```python
from build123d import *
from build123d.topology import SkipClean

# Parameters (mm, degrees)
SKETCH1_R                       = 246.38
SKETCH1_R_2                     = 59.69
BOSS_EXTRUDE1_DEPTH             = 81.28
SKETCH2_R                       = 355.6
SKETCH2_R_2                     = 246.38
BOSS_EXTRUDE2_DEPTH             = 204.47
BOSS_EXTRUDE3_START             = 381
SKETCH3_R                       = 254
BOSS_EXTRUDE3_DEPTH             = 25.4
BOSS_EXTRUDE3_DIRECTION_2_REACH = 1339.721
SKETCH4_R                       = 30.48
CUT_EXTRUDE1_DEPTH              = 38.1
SKETCH4_4_R                     = 127
CUT_EXTRUDE2_DEPTH              = 63.5
SKETCH5_R                       = 71.12
CUT_EXTRUDE3_DEPTH              = 762


with BuildPart() as part:
    # Sketch1 → Boss-Extrude1 (new body)
    with BuildSketch(Plane(origin=(0, 0, 0), x_dir=(1, 0, 0), z_dir=(0, 1, 0))):
        with BuildLine():
            Line((-127, 444.5), (-127, 332.148099))
            ThreePointArc((-127, 332.148099), (-307.958634, 177.8), (-351.148692, -56.088823))
            Line((-351.148692, -56.088823), (-448.448292, -112.264774))
            ThreePointArc((-448.448292, -112.264774), (-494.933518, -285.75), (-321.448292, -332.235226))
            Line((-321.448292, -332.235226), (-224.148692, -276.059276))
            ThreePointArc((-224.148692, -276.059276), (0, -355.6), (224.148692, -276.059276))
            Line((224.148692, -276.059276), (321.448292, -332.235226))
            ThreePointArc((321.448292, -332.235226), (494.933518, -285.75), (448.448292, -112.264774))
            Line((448.448292, -112.264774), (351.148692, -56.088823))
            ThreePointArc((351.148692, -56.088823), (307.958634, 177.8), (127, 332.148099))
            Line((127, 332.148099), (127, 444.5))
            ThreePointArc((127, 444.5), (0, 571.5), (-127, 444.5))
        make_face()
        with Locations(Location((0, 0, 0), (0, 0, 270))):
            Circle(SKETCH1_R, mode=Mode.SUBTRACT)
        with Locations(Location((0, 444.5, 0), (0, 0, 270))):
            Circle(SKETCH1_R_2, mode=Mode.SUBTRACT)
        with Locations(Location((384.948292, -222.25, 0), (0, 0, 270))):
            Circle(SKETCH1_R_2, mode=Mode.SUBTRACT)
        with Locations(Location((-384.948292, -222.25, 0), (0, 0, 270))):
            Circle(SKETCH1_R_2, mode=Mode.SUBTRACT)
    extrude(amount=BOSS_EXTRUDE1_DEPTH)

    # Sketch2 → Boss-Extrude2 (add)
    with BuildSketch(Plane(origin=(0, 81.28, 0), x_dir=(1, 0, 0), z_dir=(0, 1, 0))):
        with Locations(Location((0, 0, 0), (0, 0, 69.075168))):
            Circle(SKETCH2_R)
        with Locations(Location((0, 0, 0), (0, 0, 270))):
            Circle(SKETCH2_R_2, mode=Mode.SUBTRACT)
    extrude(amount=BOSS_EXTRUDE2_DEPTH)

    # Mirror2: part across plane


with BuildPart() as part_1:
    add(part.part)
    add(part.part.mirror(Plane.ZX.offset(285.75)))

    # Sketch3 → Boss-Extrude3 (add)
    with BuildSketch(Plane.XY.offset(BOSS_EXTRUDE3_START)):
        with Locations((0, 285.75)):
            Circle(SKETCH3_R)
    extrude(amount=BOSS_EXTRUDE3_DEPTH)

    # Sketch3 → Boss-Extrude3 direction 2 (add, up to next)
    with BuildSketch(Plane.XY.offset(BOSS_EXTRUDE3_START), mode=Mode.PRIVATE) as boss_extrude3_direction_2_sk1:
        with Locations((0, 285.75)):
            Circle(SKETCH3_R)
    boss_extrude3_direction_2_tool1 = extrude(boss_extrude3_direction_2_sk1.sketch, amount=-BOSS_EXTRUDE3_DIRECTION_2_REACH, mode=Mode.PRIVATE) - part_1.part
    add(boss_extrude3_direction_2_tool1.solids().sort_by_distance((0, 285.75, 381))[0])

    # Sketch4 → Cut-Extrude1 (cut)
    with SkipClean():  # the faces are left unmerged after this step: merging them gives an invalid solid
        with BuildSketch(Plane.XY.offset(406.4)):
            with Locations((0, 476.25)):
                Circle(SKETCH4_R)
            with Locations((164.977839, 190.5)):
                Circle(SKETCH4_R)
            with Locations((-164.977839, 190.5)):
                Circle(SKETCH4_R)
        extrude(amount=-CUT_EXTRUDE1_DEPTH, mode=Mode.SUBTRACT)

    # Sketch4_4 → Cut-Extrude2 (cut)
    with SkipClean():  # the faces are left unmerged after this step: merging them gives an invalid solid
        with BuildSketch(Plane.XY.offset(406.4)):
            with Locations((0, 285.75)):
                Circle(SKETCH4_4_R)
        extrude(amount=-CUT_EXTRUDE2_DEPTH, mode=Mode.SUBTRACT)

    # Sketch5 → Cut-Extrude3 (cut)
    with SkipClean():  # the faces are left unmerged after this step: merging them gives an invalid solid
        with BuildSketch(Plane.XY.offset(342.9)):
            with Locations((0, 285.75)):
                Circle(SKETCH5_R)
        extrude(amount=-CUT_EXTRUDE3_DEPTH, mode=Mode.SUBTRACT)


solid = part_1.part
```
Input: part model. Units: mm. Frame: model coordinates. A direction names the side the tool comes from. Coordinates: 2 decimals unless noted, no trailing zeros. Loops run counter-clockwise (first coordinate to the right, second up) from the corner with the lowest first, then second, coordinate; pieces in that order, holes last.
Q1. Section D-D, the plane x = 0. Give the number of separate pieces and of enclosed holes in the cut face, and give its area (3 significant figures).
Results are:
separate pieces: 6
enclosed holes: 0
area: 119,000 mm2
Q2. Mould query, pull axis Z, two halves, no side actions, for faces 6 (the flat face through (272.117, 40.071, 303.754)), 7 (the flat face through (-2, 0, -247)), 8 (the cylindrical face through (-421.269, 40.071, 174.882)). Classes: +Z half, -Z half, draft (parallel to the pull), parting line (faces both ways), or undercut.
Results are:
face 6: +Z half
face 7: draft
face 8: undercut
Q3. Line query: line 1 along Y through (x, z) = (0, 368); line 2 along X through (y, z) = (547, 6); line 3 along Z through (x, y) = (223, 399). Output: solid intervals per line, ascending.
Results are:
line 1: y = 31.75 to 158.75, 412.75 to 539.75
line 2: x = -355.55 to -246.31, 246.31 to 355.55
line 3: z = -276.99 to -104.76, 104.76 to 406.4
Q4. Section B-B, the plane y = 341. Return the cut outline in (x, z).
Results are:
outline: (-247.92, 254.93) arc R355.6 ccw to (-44.78, -352.77) - (-44.78, -242.28) arc R246.38 cw to (-44.78, 242.28) - (-44.78, 342.9) - (-114.35, 342.9) - (-114.35, 406.4) - (-247.92, 406.4) - close; (44.78, -352.77) arc R355.6 ccw to (247.92, 254.93) - (247.92, 406.4) - (114.35, 406.4) - (114.35, 342.9) - (44.78, 342.9) - (44.78, 242.28) arc R246.38 cw to (44.78, -242.28) - close
Q5. Contact query for flat-ended pins moving along their axis: pin 1 (6 mm diameter, centred on x = 119.5, y = 127, fed in from -Z); pin 2 (2 mm diameter, centred on y = 326, z = 191.5, fed in from +X); pin 3 (2 mm diameter, centred on y = 195, z = 160.5, fed in from -X); pin 4 (4 mm diameter, centred on x = -147, z = 200.5, fed in from -Y). Output: stop coordinate, or through.
Results are:
pin 1: stops at z = -335.97
pin 2: stops at x = 300.27
pin 3: stops at x = -317.82
pin 4: stops at y = 0
Q6. Section A-A, the plane z = 0. Return the cut outline in (x, y).
Results are:
outline: (-355.6, 0) - (-246.38, 0) - (-246.38, 571.5) - (-355.6, 571.5) - close; (246.38, 0) - (355.6, 0) - (355.6, 571.5) - (246.38, 571.5) - close
Q7. Section C-C, the plane y = 190.5. Return the cut outline in (x, z), and give its area (3 significant figures).
Results are:
outline: (-235.46, 266.47) arc R355.6 ccw (long way) to (235.46, 266.47) - (235.46, 406.4) - (195.46, 406.4) - (195.46, 368.3) - (134.5, 368.3) - (134.5, 406.4) - (84, 406.4) - (84, 342.9) - (-84, 342.9) - (-84, 406.4) - (-134.5, 406.4) - (-134.5, 368.3) - (-195.46, 368.3) - (-195.46, 406.4) - (-235.46, 406.4) - close; hole circle Ø492.76 at (0, 0)
area: 228,000 mm2
Q8. Set-up query: faces 1 (the flat face through (-273.48, 40.07, 304.54)), 2 (the flat face through (55, 231, 342.9)), 3 (the flat face through (430, 81.28, 266)), 4 (the flat face through (-127, 531, -389)), 5 (the flat face through (-434, 81.28, 266)). Return all of +Z, -Z, +X, -X, +Y, -Y with unobstructed straight access to the full face (end or side cutting, diameter ignored); none if empty.
Results are:
face 1: +Z, -Y
face 2: +Z
face 3: +Z, +X
face 4: -Z, -X, +Y, -Y
face 5: +Z, -X
